Model file for the job. Use its own axes, mm. A direction names the side the tool comes from. Round coordinates to 2 decimals unless told otherwise and drop trailing zeros. Order: outer loops, then holes, each group sorted by start corner. A loop starts at its lowest first (then second) coordinate and runs counter-clockwise, first axis right, second up. Notation, with made-up numbers: M 44.5,-9 L 87.5,-9 A27 cw 87.5,11 Z; hole C -38.75,-26 d9. An arc over 180 degrees is marked long. Return JSON: item names as keys, results as strings. Group by question number.
Item 1: Slice it at A-A on x = 0. Write the cut outline in (y, z), then the cut area to 3 significant figures.
Item 2: Slice it at B-B on y = -10.25. Write the cut outline in (x, z), then the cut area to 3 significant figures.
Item 3: Slice it at C-C on z = 3.5. Write the cut outline in (x, y).
Item 4: Probe line 1 along Y through (x, z) = (0, 4.2); line 2 along X through (y, z) = (-12.5, 4.2); line 3 along Y through (x, z) = (0, 3.25). List the from-to ranges inside material, lowest first.
Item 5: Pull direction Z, two halves, no side cores. Call faces 3 (the face through (-0.108, -0.488, 2.465)), 4 (the face through (0, -9, 3)), 5 (the face through (0, -6, 0)), 6 (the face through (0, -11, 1)): pulls with the +Z half, pulls with the -Z half, needs draft (parallel to the pull), parting line crosses it, or undercut.
Item 6: Pin check, flat tip, straight feed: pin 1 Ø1 at (y, z) = (-11, 2) entering from +X. Stop position of the tip, or through.
Item 7: Which spindle directions (+Z, -Z, +X, -X, +Y, -Y) get a long thin tool onto all of the face, cutting with end or side? Do faces 1 (the face through (2.5, -5, 2)), 2 (the face through (0, -11, 4)). Say none if no direction does.
from build123d import *

# Parameters (mm, degrees)
CROQUIS1_R              = 0.5
SALIENTE_EXTRUIR2_DEPTH = 5
CROQUIS3_W              = 3
CROQUIS3_H              = 3.5
CROQUIS3_H_2            = 3.121183209
CORTAR_EXTRUIR2_DEPTH   = 5
REDONDEO1_R             = 0.5
REDONDEO2_R             = 0.5


with BuildPart() as part:
    # Croquis1 → Saliente-Extruir2 (new body)
    with BuildSketch(Plane.XY):
        with BuildLine():
            Line((-2.5, 0), (-2.5, -12.5))
            ThreePointArc((-2.5, -12.5), (0, -15), (2.5, -12.5))
            Line((2.5, -12.5), (2.5, 0))
            ThreePointArc((2.5, 0), (0, 2.5), (-2.5, 0))
        make_face()
        Circle(CROQUIS1_R, mode=Mode.SUBTRACT)
        with Locations((0, -12.5)):
            Circle(CROQUIS1_R, mode=Mode.SUBTRACT)
    extrude(amount=SALIENTE_EXTRUIR2_DEPTH)

    # Croquis3 → Cortar-Extruir2 (cut)
    with BuildSketch(Plane(origin=(2.5, 0, 0), x_dir=(0, 0, -1), z_dir=(1, 0, 0))):
        with Locations((-2.5, -10.75)):
            Rectangle(CROQUIS3_W, CROQUIS3_H)
        with Locations((-2.5, -14.060591605)):
            Rectangle(CROQUIS3_W, CROQUIS3_H_2)
    extrude(amount=-CORTAR_EXTRUIR2_DEPTH, mode=Mode.SUBTRACT)

    # Redondeo1
    redondeo1_edges = [part.edges().sort_by_distance(p)[0] for p in [
        (-2.5, -6.25, 5),
        (0, -15, 5),
        (2.5, -6.25, 5),
        (0, 2.5, 5),
    ]]
    fillet(redondeo1_edges, radius=REDONDEO1_R)

    # Redondeo2
    redondeo2_edges = [part.edges().sort_by_distance(p)[0] for p in [
        (-2.5, -6.25, 0),
        (0, 2.5, 0),
        (2.5, -6.25, 0),
        (0, -15, 0),
    ]]
    fillet(redondeo2_edges, radius=REDONDEO2_R)


solid = part.part
Output values:
{
 "1": {"outline": "M -15,0.5 A0.5 ccw -14.5,0 L -13,0 L -13,1 L -15,1 Z; M -15,4 L -13,4 L -13,5 L -14.5,5 A0.5 ccw -15,4.5 Z; M -12,0 L -0.5,0 L -0.5,5 L -12,5 L -12,4 L -9,4 L -9,1 L -12,1 Z; M 0.5,0 L 2,0 A0.5 ccw 2.5,0.5 L 2.5,4.5 A0.5 ccw 2,5 L 0.5,5 Z", "area": "62.3 mm²"},
 "2": {"outline": "M -2.5,0.5 A0.5 ccw -2,0 L 2,0 A0.5 ccw 2.5,0.5 L 2.5,1 L -2.5,1 Z; M -2.5,4 L 2.5,4 L 2.5,4.5 A0.5 ccw 2,5 L -2,5 A0.5 ccw -2.5,4.5 Z", "area": "9.79 mm²"},
 "3": {"outline": "M -2.5,-9 L 2.5,-9 L 2.5,0 A2.5 ccw -2.5,0 Z; hole C 0,0 d1"},
 "4": {"line 1": "-15 to -13, -12 to -0.5, 0.5 to 2.5", "line 2": "-2.5 to -0.5, 0.5 to 2.5", "line 3": "-9 to -0.5, 0.5 to 2.5"},
 "5": {"face 3": "needs draft", "face 4": "undercut", "face 5": "pulls with the -Z half", "face 6": "undercut"},
 "6": {"pin 1": "through"},
 "7": {"face 1": "+Z, -Z, +X, +Y, -Y", "face 2": "+X, -X, -Y"}
}
